For this review, use the dimensioned drawing (mm, ordinates from the lowest corner) and the shaded views. A direction names the side the tool comes from. Give positions to 0.01 mm unless a question says otherwise; leave off trailing zeros. Loops run counter-clockwise (first coordinate to the right, second up) from the corner with the lowest first, then second, coordinate; pieces in that order, holes last. Notation, with made-up numbers: M -35.5,-9.75 L -5.5,-9.75 A13 ccw -5.5,-3.75 Z; hole C 52.25,-22.5 d11. An arc over 180 degrees is marked long. Use CSV: the item, a comma, the result in double quotes. Start each with the question number.
1. Take a section at A-A, the plane x = 3.5. Write out the cut boundary in (y, z).
2. Insertion check: P1, Ø1, axis at x = 4, y = 49, coming from the +Z side; P2, Ø3, axis at x = 9, y = 49, coming from the -Z side; P3, Ø5.5, axis at x = 6, z = 6, coming from the +Y side. Each pin has a flat end and moves straight along its axis. Give the tip position at first contact, or say it passes through.
3. Take a section at D-D, the plane y = 14. Write out the cut boundary in (x, z).
4. To check wall thickness, follow line 1 (Y direction, x = 2.75, z = 6); line 2 (Y direction, x = 8.75, z = 6); line 3 (Z direction, x = 6.25, y = 34.8). State the ranges of each line that lie inside material, in increasing order. Write a range as [from, to].
5. Take a section at B-B, the plane z = 6. Write out the cut boundary in (x, y), and give its area (3 significant figures).
6. The part is to be moulded in two halves that separate along X. For the marked faces 4, 5, 6 and 7, say which applies: pulls with the +X half, pulls with the -X half, needs draft (parallel to the pull), parting line crosses it, or undercut.
7. Tool access review of the marked faces 1, 2 and 3: name each direction out of +Z, -Z, +X, -X, +Y, -Y from which nothing blocks a thin tool from reaching the whole face with its end or side.
8. Take a section at C-C, the plane z = 8.5. Write out the cut boundary in (x, y), and give its area (3 significant figures).
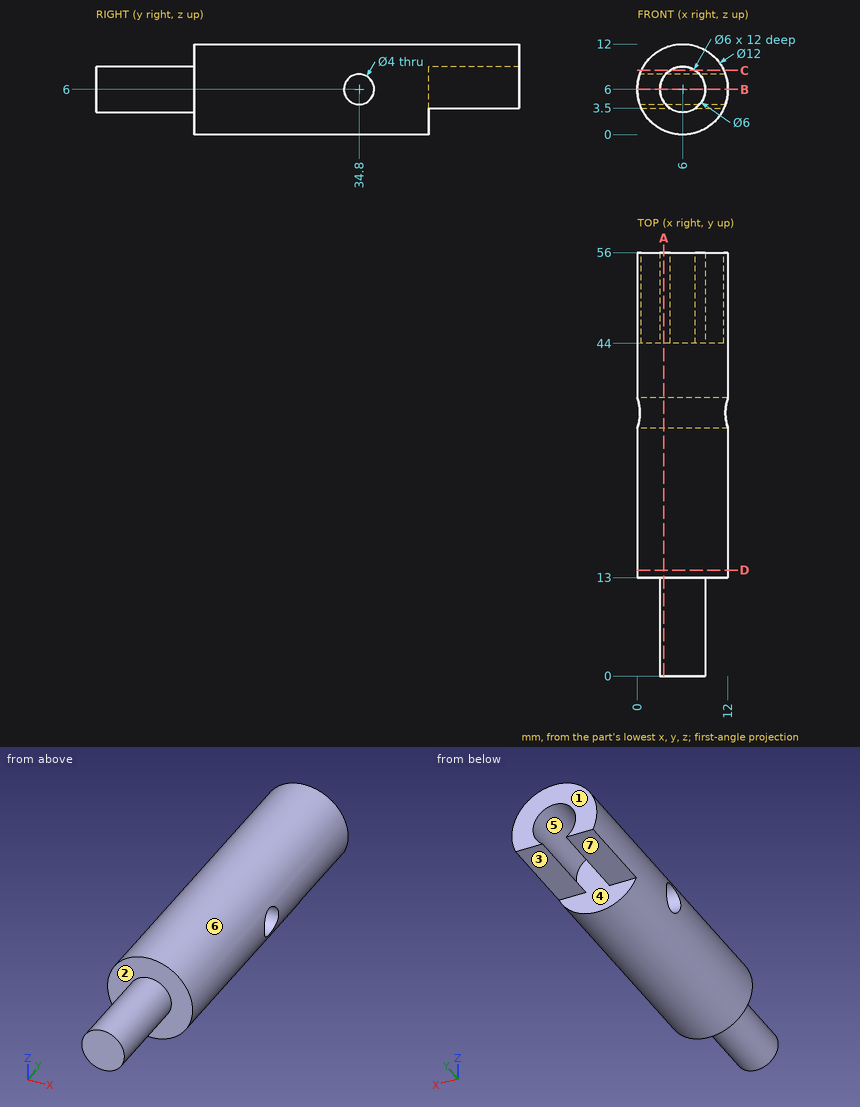
Result set:
1,outline,"M 0,4.34 L 13,4.34 L 13,0.55 L 44,0.55 L 44,3.5 L 56,3.5 L 56,4.34 L 44,4.34 L 44,7.66 L 56,7.66 L 56,11.45 L 13,11.45 L 13,7.66 L 0,7.66 Z; hole C 34.8,6 d4"
2,P1,"z = 11.81"
2,P2,"z = 3.5"
2,P3,"y = 44"
3,outline,"C 6,6 d12"
4,line 1,"[13, 32.8], [36.8, 56]"
4,line 2,"[0, 32.8], [36.8, 44]"
4,line 3,"[0.01, 4], [8, 11.99]"
5,outline,"M 0,13 L 3,13 L 3,0 L 9,0 L 9,13 L 12,13 L 12,32.8 L 0,32.8 Z; M 0,36.8 L 12,36.8 L 12,56 L 9,56 L 9,44 L 3,44 L 3,56 L 0,56 Z"
5,area,"474 mm2"
6,face 4,"undercut"
6,face 5,"undercut"
6,face 6,"parting line crosses it"
6,face 7,"needs draft"
7,face 1,"+Z, -Z, +X, -X, +Y"
7,face 2,"-Y"
7,face 3,"-Z, +X, -X, +Y"
8,outline,"M 0.55,13 L 4.34,13 L 4.34,0 L 7.66,0 L 7.66,13 L 11.45,13 L 11.45,56 L 7.66,56 L 7.66,44 L 4.34,44 L 4.34,56 L 0.55,56 Z"
8,area,"472 mm2"
